```python
from build123d import *

# Parameters (mm, degrees)
PAD_DEPTH       = 8
PAD001_DEPTH    = 10
POCKET_DEPTH    = 3
POCKET001_DEPTH = 3


with BuildPart() as part:
    # Sketch → Pad (new body)
    with BuildSketch(Plane.XY):
        with BuildLine():
            ThreePointArc((0, 30.5), (5, 35.5), (0, 40.5))
            Line((0, 40.5), (0, 45.640639))
            ThreePointArc((10.140639, 35.499973), (7.170524, 42.670505), (0, 45.640639))
            Line((10.140639, 35.499973), (10.140639, 0))
            Line((0, 0), (10.140639, 0))
            Line((0, 30.5), (0, 0))
        make_face()
    pad = extrude(amount=PAD_DEPTH)

    # Sketch001 (on Face6 of Pad) → Pad001 (join)
    with BuildSketch(Plane.XZ):
        with BuildLine():
            ThreePointArc((10.140639, 28.999961), (7.170518, 36.170482), (0, 39.14061))
            Line((0, 39.14061), (0, 33.199971))
            ThreePointArc((4.2, 28.999985), (2.969843, 31.969824), (0, 33.199971))
            Line((4.2, 23.999985), (4.2, 28.999985))
            ThreePointArc((0, 19.8), (2.969843, 21.030146), (4.2, 23.999985))
            Line((0, 19.8), (0, 8))
            Line((0, 8), (10.140639, 8))
            Line((10.140639, 8), (10.140639, 28.999961))
        make_face()
    pad001 = extrude(amount=-PAD001_DEPTH)

    # Sketch002 (on Face9 of Pad001) → Pocket (cut)
    with BuildSketch(Plane.XZ):
        Polygon((0, 16.436711), (6.55, 20.218356), (6.55, 33.218356), (0, 37), align=None)
    pocket = extrude(amount=-POCKET_DEPTH, mode=Mode.SUBTRACT)

    # Sketch003 (on Face5 of Pocket) → Pocket001 (cut)
    with BuildSketch(Plane.XY.offset(8)):
        Polygon((4.070319, 28.45), (8.140639, 35.5), (4.070319, 42.55), (0, 42.55), (0, 28.45), align=None)
    pocket001 = extrude(amount=-POCKET001_DEPTH, mode=Mode.SUBTRACT)

    # Mirrored: Pad, Pad001, Pocket, Pocket001 across Sketch V_Axis
    add(pad.mirror(Plane(origin=(0, 0, 0), x_dir=(0, 0, 1), z_dir=(1, 0, 0))))
    add(pad001.mirror(Plane(origin=(0, 0, 0), x_dir=(0, 0, 1), z_dir=(1, 0, 0))))
    add(pocket.mirror(Plane(origin=(0, 0, 0), x_dir=(0, 0, 1), z_dir=(1, 0, 0))), mode=Mode.SUBTRACT)
    add(pocket001.mirror(Plane(origin=(0, 0, 0), x_dir=(0, 0, 1), z_dir=(1, 0, 0))), mode=Mode.SUBTRACT)


solid = part.part
```
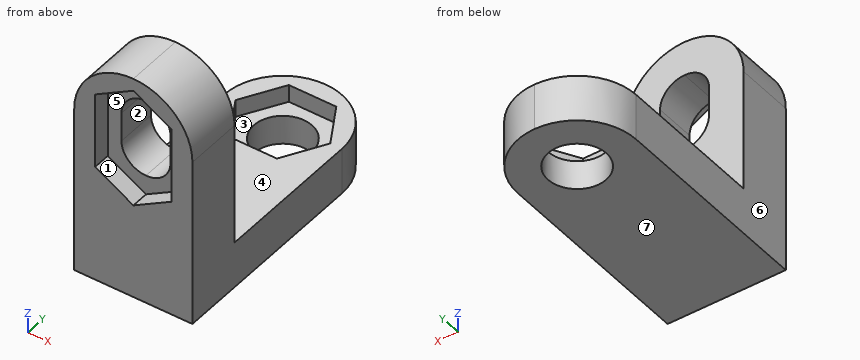
Model file for the job. Use its own axes, mm. Face numbers are marked on the shaded views. A direction names the side the tool comes from. Round coordinates to 2 decimals unless told otherwise and drop trailing zeros. Write each loop counter-clockwise with the first axis right and the second up, starting at its lowest first coordinate (ties: lowest second). Pieces come first, ordered by that corner, then holes. Notation, with made-up numbers: (-38.75, 69.5) - (0.25, 69.5) arc R19 ccw to (0.25, 74.5) - close; hole circle Ø11 at (46, -6). An arc over 180 degrees is marked (long way). One line per item, written item: value.
(1) Drop flat-ended pins along their axis: P1, Ø3, axis at x = -2, y = 8, coming from the +Z side; P2, Ø6, axis at x = 1.5, z = 22, coming from the +Y side; P3, Ø0.9, axis at x = -2, z = 6.5, coming from the +Y side; P4, Ø1, axis at x = 2, z = 27.5, coming from the +Y side. Give the stop position or say it passes through.
Values follow:
P1: stops at z = 39.13
P2: stops at y = 10
P3: stops at y = 45.52
P4: passes through
(2) Cut at A-A, the plane z = 6.5. Give the cut face in (x, y).
Values follow:
outline: (-10.14, 0) - (10.14, 0) - (10.14, 35.5) arc R10.14 ccw to (-10.14, 35.5) - close; hole (-8.14, 35.5) - (-4.07, 28.45) - (4.07, 28.45) - (8.14, 35.5) - (4.07, 42.55) - (-4.07, 42.55) - close
(3) 3-axis set-ups, long thin cutter, end or side, ignore diameter. For the marked faces 1, 2, 3 and 4: which of +Z, -Z, +X, -X, +Y, -Y reach the whole face in a straight line?
Values follow:
face 1: -Y
face 2: +Y, -Y
face 3: +Z
face 4: +Z, +X, -X, +Y
(4) Cut at B-B, the plane y = 8.5. Give the cut face in (x, z).
Values follow:
outline: (-10.14, 0) - (10.14, 0) - (10.14, 29) arc R10.14 ccw to (-10.14, 29) - close; hole (-4.2, 24) arc R4.2 ccw to (4.2, 24) - (4.2, 29) arc R4.2 ccw to (0, 33.2) arc R4.2 ccw to (-4.2, 29) - close
(5) Two-plate mould, pull along Z, no slides. Class the marked faces 5, 6 and 7: pulls with the +Z half, pulls with the -Z half, needs draft (parallel to the pull), parting line crosses it, or undercut.
Values follow:
face 5: undercut
face 6: needs draft
face 7: pulls with the -Z half
(6) Wall check: probe 1 along Y at (x, z) = (0, 3.35); probe 2 along X at (y, z) = (9, 29); probe 3 along X at (y, z) = (35.5, 1.4). Give the ranges that are in metal, low to high.
Values follow:
probe 1: y = 0 to 30.5, 40.5 to 45.64
probe 2: x = -10.14 to -4.2, 4.2 to 10.14
probe 3: x = -10.14 to -5, 5 to 10.14
(7) Cut at C-C, the plane x = -2.5. Give the cut face in (y, z), plus the area to 3 significant figures.
Values follow:
outline: (0, 0) - (31.17, 0) - (31.17, 5) - (28.45, 5) - (28.45, 8) - (10, 8) - (10, 20.63) - (3, 20.63) - (3, 17.88) - (0, 17.88) - close; (0, 35.56) - (3, 35.56) - (3, 32.37) - (10, 32.37) - (10, 38.83) - (0, 38.83) - close; (39.83, 0) - (45.33, 0) - (45.33, 8) - (42.55, 8) - (42.55, 5) - (39.83, 5) - close
area: 450 mm²
(8) Cut at D-D, the plane z = 30.5. Give the cut face in (x, y), plus the area to 3 significant figures.
Values follow:
outline: (-10.03, 0) - (-6.55, 0) - (-6.55, 3) - (-3.92, 3) - (-3.92, 10) - (-10.03, 10) - close; (3.92, 3) - (6.55, 3) - (6.55, 0) - (10.03, 0) - (10.03, 10) - (3.92, 10) - close
area: 106 mm²
